```python
from build123d import *

# Parameters (mm, degrees)
BOSS_EXTRUDE1_DEPTH = 50
SKETCH2_R           = 60
CUT_EXTRUDE1_DEPTH  = 13
SKETCH3_R           = 10
CUT_EXTRUDE2_DEPTH  = 50
SKETCH4_R           = 2
BOSS_EXTRUDE2_DEPTH = 13
CUT_EXTRUDE3_DEPTH  = 30
SKETCH6_R           = 6
BOSS_EXTRUDE4_DEPTH = 3
SKETCH7_R           = 30
CUT_EXTRUDE4_DEPTH  = 40
CUT_EXTRUDE5_DEPTH  = 25


with BuildPart() as part:
    # Sketch1 → Boss-Extrude1 (new body)
    with BuildSketch(Plane(origin=(0, 0, 0), x_dir=(1, 0, 0), z_dir=(0, 1, 0))):
        with BuildLine():
            Line((-57.148676171, 55.458248473), (62.851323829, 55.458248473))
            ThreePointArc((62.851323829, 55.458248473), (69.922391641, 52.529316284), (72.851323829, 45.458248473))
            Line((72.851323829, 45.458248473), (72.851323829, -74.541751527))
            ThreePointArc((72.851323829, -74.541751527), (69.922391641, -81.612819339), (62.851323829, -84.541751527))
            Line((62.851323829, -84.541751527), (-57.148676171, -84.541751527))
            ThreePointArc((-57.148676171, -84.541751527), (-64.219743983, -81.612819339), (-67.148676171, -74.541751527))
            Line((-67.148676171, -74.541751527), (-67.148676171, 45.458248473))
            ThreePointArc((-67.148676171, 45.458248473), (-64.219743983, 52.529316284), (-57.148676171, 55.458248473))
        make_face()
    extrude(amount=BOSS_EXTRUDE1_DEPTH)

    # Sketch2 → Cut-Extrude1 (cut)
    with BuildSketch(Plane(origin=(0, 50, 0), x_dir=(1, 0, 0), z_dir=(0, 1, 0))):
        with Locations(Location((2.851323829, -14.541751527, 0), (0, 0, 270))):
            Circle(SKETCH2_R)
    extrude(amount=-CUT_EXTRUDE1_DEPTH, mode=Mode.SUBTRACT)

    # Sketch3 → Cut-Extrude2 (cut)
    with BuildSketch(Plane(origin=(0, 37, 0), x_dir=(1, 0, 0), z_dir=(0, 1, 0))):
        with Locations(Location((2.851323829, -14.541751527, 0), (0, 0, 270))):
            Circle(SKETCH3_R)
    extrude(amount=-CUT_EXTRUDE2_DEPTH, mode=Mode.SUBTRACT)

    # Sketch4 → Boss-Extrude2 (add)
    with BuildSketch(Plane(origin=(0, 37, 0), x_dir=(1, 0, 0), z_dir=(0, 1, 0))):
        with Locations(Location((2.851323829, 33.458248473, 0), (0, 0, 90))):
            Circle(SKETCH4_R)
        with Locations(Location((36.792449326, 19.399373969, 0), (0, 0, 90))):
            Circle(SKETCH4_R)
        with Locations(Location((50.851323829, -14.541751527, 0), (0, 0, 90))):
            Circle(SKETCH4_R)
        with Locations(Location((36.792449326, -48.482877024, 0), (0, 0, 90))):
            Circle(SKETCH4_R)
        with Locations(Location((2.851323829, -62.541751527, 0), (0, 0, 90))):
            Circle(SKETCH4_R)
        with Locations(Location((-31.089801668, -48.482877024, 0), (0, 0, 90))):
            Circle(SKETCH4_R)
        with Locations(Location((-45.148676171, -14.541751527, 0), (0, 0, 90))):
            Circle(SKETCH4_R)
        with Locations(Location((-31.089801668, 19.399373969, 0), (0, 0, 90))):
            Circle(SKETCH4_R)
    extrude(amount=BOSS_EXTRUDE2_DEPTH)

    # Sketch5 → Cut-Extrude3 (cut)
    with BuildSketch(Plane.XZ):
        with BuildLine():
            Line((-37.148676171, 64.541751527), (42.851323829, 64.541751527))
            ThreePointArc((42.851323829, 64.541751527), (49.922391641, 61.612819339), (52.851323829, 54.541751527))
            Line((52.851323829, 54.541751527), (52.851323829, -25.458248473))
            ThreePointArc((52.851323829, -25.458248473), (49.922391641, -32.529316284), (42.851323829, -35.458248473))
            Line((42.851323829, -35.458248473), (-37.148676171, -35.458248473))
            ThreePointArc((-37.148676171, -35.458248473), (-44.219743983, -32.529316284), (-47.148676171, -25.458248473))
            Line((-47.148676171, -25.458248473), (-47.148676171, 54.541751527))
            ThreePointArc((-47.148676171, 54.541751527), (-44.219743983, 61.612819339), (-37.148676171, 64.541751527))
        make_face()
    extrude(amount=-CUT_EXTRUDE3_DEPTH, mode=Mode.SUBTRACT)

    # Sketch6 → Boss-Extrude4 (add)
    with BuildSketch(Plane.XZ):
        with Locations(Location((-57.148676171, 74.541751527, 0), (0, 0, 90))):
            Circle(SKETCH6_R)
        with Locations(Location((62.851323829, 74.541751527, 0), (0, 0, 90))):
            Circle(SKETCH6_R)
        with Locations(Location((62.851323829, -45.458248473, 0), (0, 0, 90))):
            Circle(SKETCH6_R)
        with Locations(Location((-57.148676171, -45.458248473, 0), (0, 0, 90))):
            Circle(SKETCH6_R)
    extrude(amount=BOSS_EXTRUDE4_DEPTH)

    # Sketch7 → Cut-Extrude4 (cut)
    with BuildSketch(Plane(origin=(0, 37, 0), x_dir=(1, 0, 0), z_dir=(0, 1, 0))):
        with Locations(Location((2.851323829, -14.541751527, 0), (0, 0, 270))):
            Circle(SKETCH7_R)
    extrude(amount=-CUT_EXTRUDE4_DEPTH, mode=Mode.SUBTRACT)

    # Sketch8 → Cut-Extrude5 (cut)
    with BuildSketch(Plane.ZY.offset(67.148676171)):
        with BuildLine():
            Line((-5.458248473, 0), (34.541751527, 0))
            Line((34.541751527, 0), (34.541751527, 12))
            ThreePointArc((34.541751527, 12), (33.663071871, 14.121320344), (31.541751527, 15))
            Line((31.541751527, 15), (-2.458248473, 15))
            ThreePointArc((-2.458248473, 15), (-4.579568816, 14.121320344), (-5.458248473, 12))
            Line((-5.458248473, 12), (-5.458248473, 0))
        make_face()
    extrude(amount=-CUT_EXTRUDE5_DEPTH, mode=Mode.SUBTRACT)


solid = part.part
```
Verification items for the finished model (mm, model axes). A direction names the side the tool comes from. Coordinates: 2 decimals unless noted, no trailing zeros. Order: outer loops, then holes, each group sorted by start corner. A loop starts at its lowest first (then second) coordinate and runs counter-clockwise, first axis right, second up. Notation, with made-up numbers: (-39, 31) -> (-7, 31) arc R20 ccw to (-7, 36) -> close; hole circle Ø3 at (57, 1.5). An arc over 180 degrees is marked (long way). Answer as CSV lines item,"result". Start each with the question number.
1) Cross-section at D-D, the plane z = 10.5. Record the boundary of the cut face in (x, y), then the cut area to 3 significant figures.
2) Release check for a two-part mould opening along X. For faces 4 (the face through (30.4, 37, 27)), 5 (the face through (69.84, 24.65, -52.61)), 6 (the face through (-57, 15, 15)) record: released by +X, released by -X, zero draft, split by the parting line, or undercut.
3) Cross-section at B-B, the plane x = 12.5. Record the boundary of the cut face in (y, z), then the cut area to 3 significant figures.
4) Cross-section at C-C, the plane y = 39. Give the number of separate pieces and of enclosed holes in the cut face, then the cut area to 3 significant figures.
5) Gauge pin test, flat ends, axial feed: pin 1 Ø4 at (x, z) = (-43.5, -3.5) entering from +Y; pin 2 Ø16 at (x, z) = (-61.5, 7) entering from -Y. Record the tip position at first contact, or that the pin passes through.
6) Material ranges on L1, parallel to X at y = 18, z = -8; L2, parallel to Z at x = 17, y = 8.5; L3, parallel to Z at x = -30.5, y = 40.5, recorded low to high. Write a range as [from, to].
7) Cross-section at A-A, the plane y = 17. Record the boundary of the cut face in (x, z), then the cut area to 3 significant figures.
8) Set-up check for faces 1 (the face through (-57, 6, -5.458)), 2 (the face through (-44.14, 14.79, -32.61)), 3 (the face through (3.617, 43.409, -35.306)): record each of +Z, -Z, +X, -X, +Y, -Y from which the full face is reachable in a straight line by a thin tool's end or side.
Conclusion:
1,outline,"(-67.15, 15) -> (-47.15, 15) -> (-47.15, 30) -> (-26.88, 30) -> (-26.88, 37) -> (-57.01, 37) -> (-57.01, 50) -> (-67.15, 50) -> close; (32.58, 30) -> (52.85, 30) -> (52.85, 0) -> (72.85, 0) -> (72.85, 50) -> (62.72, 50) -> (62.72, 37) -> (32.58, 37) -> close"
1,area,"1,730 mm²"
2,face 4,"undercut"
2,face 5,"released by +X"
2,face 6,"zero draft"
3,outline,"(0, -55.46) -> (50, -55.46) -> (50, -44.68) -> (37, -44.68) -> (37, -13.86) -> (30, -13.86) -> (30, -35.46) -> (0, -35.46) -> close; (0, 64.54) -> (30, 64.54) -> (30, 42.95) -> (37, 42.95) -> (37, 73.76) -> (50, 73.76) -> (50, 84.54) -> (0, 84.54) -> close"
3,area,"2,060 mm²"
4,separate pieces,"9"
4,enclosed holes,"1"
4,area,"8,300 mm²"
5,pin 1,"stops at y = 37"
5,pin 2,"stops at y = 15"
6,L1,"x = [-67.15, -47.15], [52.85, 72.85]"
6,L2,"z = [-55.46, -35.46], [64.54, 84.54]"
6,L3,"z = [-55.46, -35.33], [-21.31, -17.49], [46.57, 50.39], [64.42, 84.54]"
7,outline,"(-67.15, -45.46) arc R10 ccw to (-57.15, -55.46) -> (62.85, -55.46) arc R10 ccw to (72.85, -45.46) -> (72.85, 74.54) arc R10 ccw to (62.85, 84.54) -> (-57.15, 84.54) arc R10 ccw to (-67.15, 74.54) -> close; hole (-47.15, -25.46) arc R10 ccw to (-37.15, -35.46) -> (42.85, -35.46) arc R10 ccw to (52.85, -25.46) -> (52.85, 54.54) arc R10 ccw to (42.85, 64.54) -> (-37.15, 64.54) arc R10 ccw to (-47.15, 54.54) -> close"
7,area,"9,600 mm²"
8,face 1,"-X, -Y"
8,face 2,"-Y"
8,face 3,"+Y"
